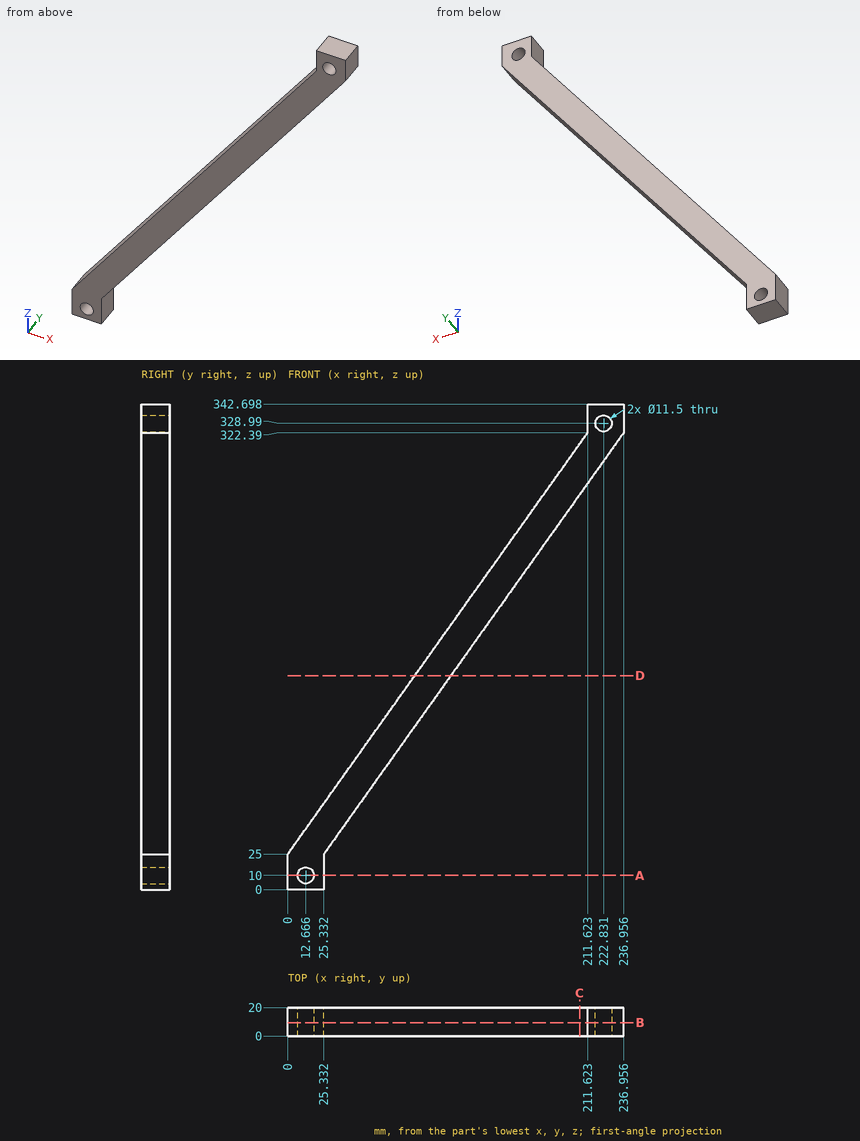
Design review of the part shown in the three views and the two pictorial views. Dimensions are in mm from the part's minimum x, y and z. Coordinates: 2 decimals unless noted, no trailing zeros. Order: outer loops, then holes, each group sorted by start corner. A loop starts at its lowest first (then second) coordinate and runs counter-clockwise, first axis right, second up. Notation, with made-up numbers: (-16.5, 73.25) - (-9.5, 73.25) arc R20 cw to (-9.5, 106.25) - close; hole circle Ø9 at (-39, -3.75). An arc over 180 degrees is marked (long way). One line per question, with ' | ' between items.
Q1. To check wall thickness, follow line 1 along X through (y, z) = (4.5, 10); line 2 along X through (y, z) = (9.25, 248); line 3 along X through (y, z) = (7.5, 146) (1 decimal). State the ranges of each line that lie inside material, in increasing order.
Answer key:
line 1: x = 0 to 6.92, 18.42 to 25.33 | line 2: x = 158.69 to 184.02 | line 3: x = 86.1 to 111.4
Q2. Consider section C-C, the plane x = 206. Give the boundary of the cut face in (y, z), then the cut area to 3 significant figures.
Answer key:
outline: (0, 278.89) - (20, 278.89) - (20, 314.49) - (0, 314.49) - close | area: 712 mm2
Q3. Consider section B-B, the plane y = 9.5. Give the number of separate pieces and of enclosed holes in the cut face, then the cut area to 3 significant figures.
Answer key:
separate pieces: 1 | enclosed holes: 2 | area: 8,470 mm2
Q4. Consider section A-A, the plane z = 10. Give the boundary of the cut face in (x, y), then the cut area to 3 significant figures.
Answer key:
outline: (0, 0) - (6.92, 0) - (6.92, 20) - (0, 20) - close; (18.42, 0) - (25.33, 0) - (25.33, 20) - (18.42, 20) - close | area: 277 mm2
Q5. Consider section D-D, the plane z = 151. Give the boundary of the cut face in (x, y) (1 decimal).
Answer key:
outline: (89.7, 0) - (115, 0) - (115, 20) - (89.7, 20) - close
Q6. Clearance check with flat-ended pins moving along their axes: pin 1 Ø12 at (x, y) = (163, 5) entering from +Z; pin 2 Ø7 at (x, z) = (222.83, 328.99) entering from -Y; pin 3 Ø18.5 at (x, z) = (12.67, 10) entering from +Y; pin 4 Ø5 at (y, z) = (8, 230) entering from -X. State where each tip first meets the part, or that it passes through.
Answer key:
pin 1: stops at z = 262.49 | pin 2: passes through | pin 3: stops at y = 20 | pin 4: stops at x = 144.1
